The listing builds one solid part. Answer for the finished solid, in the listing's coordinates (mm). A direction names the side the tool comes from. Give positions to 0.01 mm unless a question says otherwise; leave off trailing zeros. Write each loop counter-clockwise with the first axis right and the second up, starting at its lowest first coordinate (ties: lowest second). Pieces come first, ordered by that corner, then holes. Notation, with made-up numbers: (41, -6) -> (91, -6) arc R31 ccw to (91, 31) -> close; hole circle Ø10 at (83.5, -1). An arc over 180 degrees is marked (long way). One line per question, with ' | ' between items.
from build123d import *

# Parameters (mm, degrees)
IZIM1_R                     = 19
Y_KSEKLIK_EKSTR_ZYON1_DEPTH = 13
IZIM2_R                     = 2
KES_EKSTR_ZYON1_DEPTH       = 10
IZIM3_R                     = 7
Y_KSEKLIK_EKSTR_ZYON2_DEPTH = 3.5
IZIM4_R                     = 3
IZIM4_R_2                   = 2
Y_KSEKLIK_EKSTR_ZYON3_DEPTH = 17


with BuildPart() as part:
    # Çizim1 → Yükseklik-Ekstrüzyon1 (new body)
    with BuildSketch(Plane(origin=(0, 0, 0), x_dir=(1, 0, 0), z_dir=(0, 1, 0))):
        Circle(IZIM1_R)
    extrude(amount=-Y_KSEKLIK_EKSTR_ZYON1_DEPTH)

    # Çizim2 → Kes-Ekstrüzyon1 (cut)
    with BuildSketch(Plane(origin=(0, 0, 0), x_dir=(1, 0, 0), z_dir=(0, 1, 0))):
        with Locations((-15.5, 0)):
            Circle(IZIM2_R)
        with Locations((15.5, 0)):
            Circle(IZIM2_R)
    extrude(amount=-KES_EKSTR_ZYON1_DEPTH, mode=Mode.SUBTRACT)

    # Çizim3 → Yükseklik-Ekstrüzyon2 (add)
    with BuildSketch(Plane(origin=(0, 0, 0), x_dir=(1, 0, 0), z_dir=(0, 1, 0))):
        Circle(IZIM3_R)
    extrude(amount=Y_KSEKLIK_EKSTR_ZYON2_DEPTH)

    # Çizim4 → Yükseklik-Ekstrüzyon3 (add)
    with BuildSketch(Plane(origin=(0, 3.5, 0), x_dir=(1, 0, 0), z_dir=(0, 1, 0))):
        Circle(IZIM4_R)
        Circle(IZIM4_R_2, mode=Mode.SUBTRACT)
    extrude(amount=Y_KSEKLIK_EKSTR_ZYON3_DEPTH)


solid = part.part
Item 1: Find section D-D (x = 15). Write down the section's boundary in (y, z), then the cut area to 3 significant figures.
Answers below:
outline: (-13, -11.66) -> (0, -11.66) -> (0, -1.94) -> (-10, -1.94) -> (-10, 1.94) -> (0, 1.94) -> (0, 11.66) -> (-13, 11.66) -> close | area: 264 mm²
Item 2: Consider line 1 (X direction, y = -4, z = 0); line 2 (Z direction, x = 0, y = 12.5). Determine where each line is inside the solid, lowest interval first. Write a range as [from, to].
Answers below:
line 1: [-19, -17.5], [-13.5, 13.5], [17.5, 19] | line 2: [-3, -2], [2, 3]
Item 3: Find section A-A (z = -5). Write down the section's boundary in (x, y), then the cut area to 3 significant figures.
Answers below:
outline: (-18.33, -13) -> (18.33, -13) -> (18.33, 0) -> (4.9, 0) -> (4.9, 3.5) -> (-4.9, 3.5) -> (-4.9, 0) -> (-18.33, 0) -> close | area: 511 mm²
Item 4: Flat-ended cylindrical pins translate along their axes: pin 1 (4.5 mm diameter, centred on x = 16, z = 0.5, fed in from +Y); pin 2 (12 mm diameter, centred on x = -15, y = -6, fed in from -Z); pin 3 (8 mm diameter, centred on y = -6.5, z = -14.5, fed in from -X). Find the tip coordinate at first contact, or state that the pin passes through.
Answers below:
pin 1: y = 0 | pin 2: z = -16.73 | pin 3: x = -15.84
Item 5: Find section B-B (y = 14.5). Write down the section's boundary in (x, z).
Answers below:
outline: circle Ø6 at (0, 0); hole circle Ø4 at (0, 0)
Item 6: A tool of negligible diameter and unlimited length cuts with its end or side. For faces 4 (the face through (1, 20.5, 2)), 5 (the face through (0, 3.5, 0)), from which of +Z, -Z, +X, -X, +Y, -Y can it reach the whole face along a straight path? Write none if from no direction.
Answers below:
face 4: +Z, -Z, +X, -X, +Y | face 5: +Y
Item 7: Find section C-C (y = 2.5). Write down the section's boundary in (x, z), then the cut area to 3 significant figures.
Answers below:
outline: circle Ø14 at (0, 0) | area: 154 mm²
Item 8: Determine the mould class of faces 1 (the face through (-3, 12, 0)), 2 (the face through (8, 0, 0)), 3 (the face through (15, -10, 0)) for opening direction Z: pulls with the +Z half, pulls with the -Z half, needs draft (parallel to the pull), parting line crosses it, or undercut.
Answers below:
face 1: parting line crosses it | face 2: needs draft | face 3: undercut
